Can you work these out from the model? Positions are in its coordinate system, mm. A direction names the side the tool comes from. Give positions to 0.01 mm unless a question says otherwise; leave off trailing zeros. Loops run counter-clockwise (first coordinate to the right, second up) from the corner with the lowest first, then second, coordinate; pieces in that order, holes last. Notation, with made-up numbers: M 48,31.5 L 78,31.5 A18 cw 78,56.5 Z; hole C -12.75,66.5 d5. An arc over 180 degrees is marked long. Put each result on its own line as item: value. Start each with the question number.
1) For faces 1 (the flat face through (-309, 110, 19.05)), 2 (the flat face through (0, 110, 361)), which set-ups out of +Z, -Z, +X, -X, +Y, -Y let a thin tool reach every point of the face, with its end or its side?
2) Imagine slicing it at C-C (y = 131). Write out the boundary of the cut face in (x, z).
3) Imagine slicing it at A-A (z = 396). Write out the boundary of the cut face in (x, y), then the cut area to 3 significant figures.
4) If we mould it in two halves opening along Z, with no side actions, what happens to faces 3 (the flat face through (-301, 110, 711.2)), 4 (the flat face through (-590.55, 110, 273)), 5 (the flat face through (-609.6, 110, 361))? For each: +Z half, -Z half, draft (parallel to the pull), parting line (faces both ways), or undercut.
5) Imagine slicing it at B-B (x = -171.5). Write out the boundary of the cut face in (y, z), then the cut area to 4 significant figures.
6) Please list where these lines run through material, in increasing order: line 1 along Z through (x, y) = (-307, 140.5); line 2 along X through (y, z) = (162, 389). Write a range as from..to.
from build123d import *

# Parameters (mm, degrees)
F0_W     = 222.25
F0_H     = 711.2
F1_DEPTH = 609.6
F2_W     = 571.5
F2_H     = 514.35
F3_DEPTH = 285.75
F4_W     = 571.5
F4_H     = 63.5
F5_DEPTH = 158.75


with BuildPart() as f1:
    # F0 (on Right) → F1 (new body)
    with BuildSketch(Plane.YZ):
        with Locations((111.125, 355.6)):
            Rectangle(F0_W, F0_H)
    extrude(amount=-F1_DEPTH)

    # F2 (on face) → F3 (cut)
    with BuildSketch(Plane.XZ):
        with Locations((-304.8, 276.225)):
            Rectangle(F2_W, F2_H)
    extrude(amount=-F3_DEPTH, mode=Mode.SUBTRACT)

    # F4 (on face) → F5 (cut)
    with BuildSketch(Plane(origin=(0, 0, 533.4), x_dir=(1, 0, 0), z_dir=(0, 0, -1))):
        with Locations((-304.8, -254)):
            Rectangle(F4_W, F4_H)
    extrude(amount=-F5_DEPTH, mode=Mode.SUBTRACT)


solid = f1.part
Recorded:
1. face 1: +Y, -Y
1. face 2: +Z, -Z, +X, +Y, -Y
2. outline: M -609.6,0 L 0,0 L 0,711.2 L -609.6,711.2 Z; hole M -590.55,19.05 L -19.05,19.05 L -19.05,533.4 L -590.55,533.4 Z
3. outline: M -609.6,0 L -590.55,0 L -590.55,222.25 L -609.6,222.25 Z; M -19.05,0 L 0,0 L 0,222.25 L -19.05,222.25 Z
3. area: 8,470 mm²
4. face 3: +Z half
4. face 4: undercut
4. face 5: draft
5. outline: M 0,0 L 222.25,0 L 222.25,19.05 L 0,19.05 Z; M 0,533.4 L 222.25,533.4 L 222.25,711.2 L 0,711.2 Z
5. area: 43,750 mm²
6. line 1: 0..19.05, 533.4..711.2
6. line 2: -609.6..-590.55, -19.05..0
